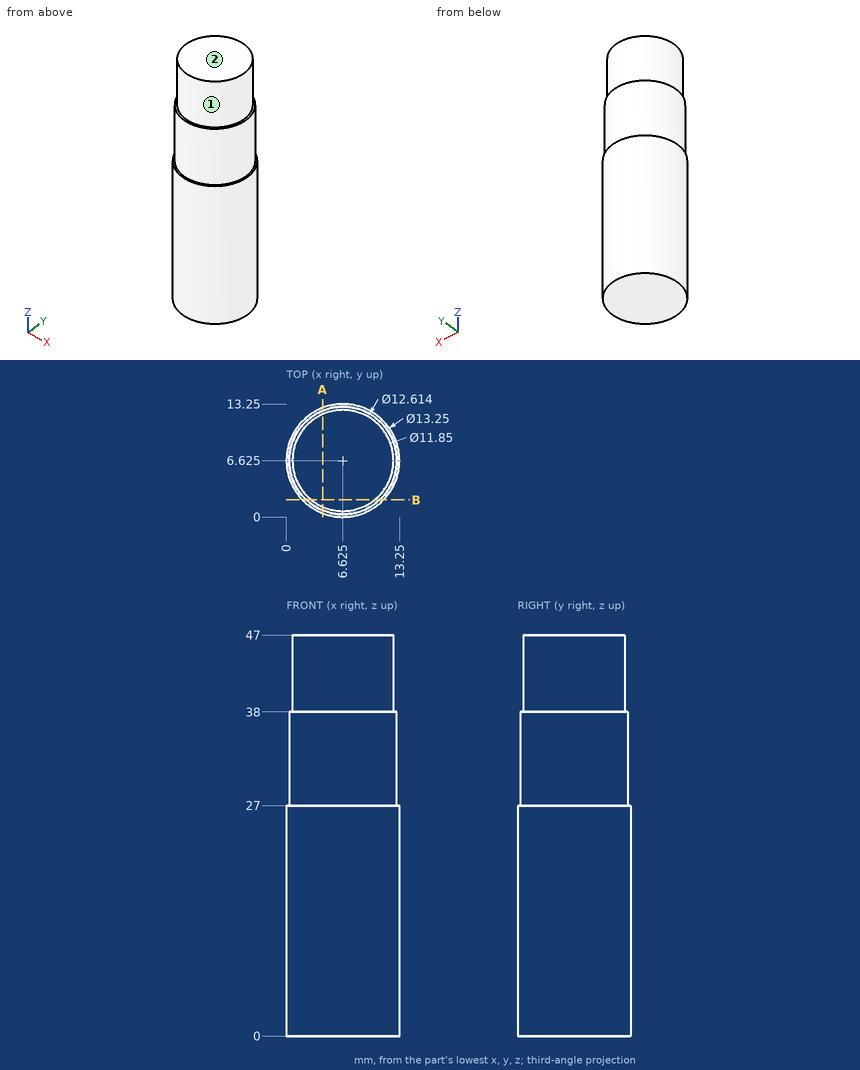
Input: dimensioned drawing with shaded views. Units: mm. Origin: part minimum x, y, z. A direction names the side the tool comes from. Give positions to 0.01 mm unless a question says otherwise; leave off trailing zeros. Write each loop counter-clockwise with the first axis right and the second up, starting at its lowest first coordinate (ties: lowest second). Pieces come first, ordered by that corner, then holes. Notation, with made-up numbers: (70.25, 85.25) - (86.25, 85.25) arc R17 ccw to (86.25, 115.25) - close; hole circle Ø10 at (44, 67). An arc over 180 degrees is marked (long way). One line per item, written item: value. Start each with the question number.
Q1. Section query B-B, the plane y = 2. Return the cut outline in (x, z), then the cut area to 3 significant figures.
Q2. Material intervals for probe 1 along X at (y, z) = (6.5, 42.5); probe 2 along Y at (x, z) = (6.75, 36), sorted ascending. Write a range as from..to.
Q3. Section query A-A, the plane x = 4.25. Return the cut outline in (y, z).
Q4. Set-up query: the marked faces 1 and 2. Return all of +Z, -Z, +X, -X, +Y, -Y with unobstructed straight access to the full face (end or side cutting, diameter ignored); none if empty.
Q5. First-contact query: pin 1 Ø5 at (y, z) = (10, 26) entering from -X. Flat tip, straight axial feed; report the tip coordinate or a pass-through.
Answer:
1. outline: (1.88, 0) - (11.37, 0) - (11.37, 27) - (10.91, 27) - (10.91, 38) - (10.33, 38) - (10.33, 47) - (2.92, 47) - (2.92, 38) - (2.34, 38) - (2.34, 27) - (1.88, 27) - close
1. area: 417 mm2
2. probe 1: x = 0.7..12.55
2. probe 2: y = 0.32..12.93
3. outline: (0.44, 0) - (12.81, 0) - (12.81, 27) - (12.47, 27) - (12.47, 38) - (12.05, 38) - (12.05, 47) - (1.2, 47) - (1.2, 38) - (0.78, 38) - (0.78, 27) - (0.44, 27) - close
4. face 1: +Z
4. face 2: +Z, +X, -X, +Y, -Y
5. pin 1: stops at x = 0.06
